Read the model definition and answer for the solid it produces. Units are mm, in the model's axes. Coordinates: 2 decimals unless noted, no trailing zeros. Write each loop counter-clockwise with the first axis right and the second up, starting at its lowest first coordinate (ties: lowest second). Pieces come first, ordered by that corner, then holes. Notation, with made-up numbers: (3.25, 82) - (57.25, 82) arc R9 ccw to (57.25, 93) - close; hole circle Ø9 at (-26, 22.5). An arc over 180 degrees is marked (long way). Return JSON: item names as keys, results as strings.
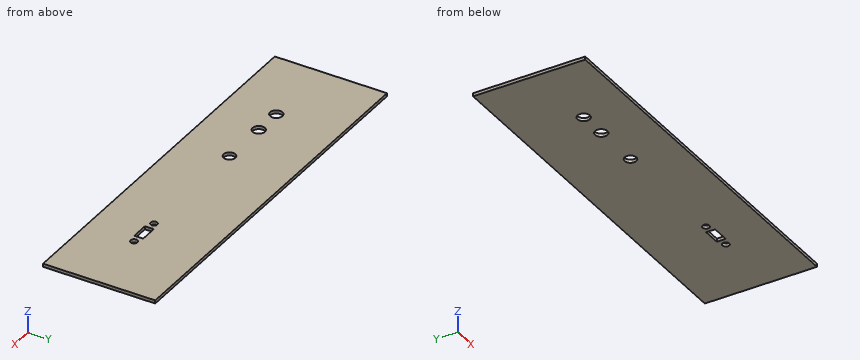
```python
from build123d import *

# Parameters (mm, degrees)
SKETCH_W      = 198
SKETCH_H      = 58
PAD_DEPTH     = 1.65
SKETCH001_R   = 1.75
SKETCH001_R_2 = 3
SKETCH001_R_3 = 3.175
SKETCH001_W   = 9.1
SKETCH001_H   = 4.6
POCKET_DEPTH  = 5


with BuildPart() as part:
    # Sketch → Pad (new body)
    with BuildSketch(Plane.XY):
        with Locations((99, 29)):
            Rectangle(SKETCH_W, SKETCH_H)
    extrude(amount=PAD_DEPTH)

    # Sketch001 (on Face6 of Pad) → Pocket (cut)
    with BuildSketch(Plane.XY.offset(1.65)):
        with Locations((144.5, 25)):
            Circle(SKETCH001_R)
        with Locations((161.5, 25)):
            Circle(SKETCH001_R)
        with Locations((80, 25)):
            Circle(SKETCH001_R_2)
        with Locations((40, 25)):
            Circle(SKETCH001_R_3)
        with Locations((55, 25)):
            Circle(SKETCH001_R_3)
        with Locations((153, 25)):
            Rectangle(SKETCH001_W, SKETCH001_H)
    extrude(amount=-POCKET_DEPTH, mode=Mode.SUBTRACT)


solid = part.part
```
(1) A cutting plane is placed at B-B (y = 25). Determine the outline of the cut face in (x, z) (3 decimals), and give its area (3 significant figures).
Answer:
{"outline": "(0, 0) - (36.825, 0) - (36.825, 1.65) - (0, 1.65) - close; (43.175, 0) - (51.825, 0) - (51.825, 1.65) - (43.175, 1.65) - close; (58.175, 0) - (77, 0) - (77, 1.65) - (58.175, 1.65) - close; (83, 0) - (142.75, 0) - (142.75, 1.65) - (83, 1.65) - close; (146.25, 0) - (148.45, 0) - (148.45, 1.65) - (146.25, 1.65) - close; (157.55, 0) - (159.75, 0) - (159.75, 1.65) - (157.55, 1.65) - close; (163.25, 0) - (198, 0) - (198, 1.65) - (163.25, 1.65) - close", "area": "269 mm²"}
(2) A flat-ended cylindrical pin translates along its axis: P1, Ø9.5, axis at x = 80, y = 25, coming from the +Z side. Find the tip coordinate at first contact, or state that the pin passes through.
Answer:
{"P1": "z = 1.65"}
(3) A cutting plane is placed at A-A (x = 55). Determine the outline of the cut face in (y, z) (3 decimals), and give its area (3 significant figures).
Answer:
{"outline": "(0, 0) - (21.825, 0) - (21.825, 1.65) - (0, 1.65) - close; (28.175, 0) - (58, 0) - (58, 1.65) - (28.175, 1.65) - close", "area": "85.2 mm²"}
(4) A cutting plane is placed at C-C (x = 144.5). Determine the outline of the cut face in (y, z).
Answer:
{"outline": "(0, 0) - (23.25, 0) - (23.25, 1.65) - (0, 1.65) - close; (26.75, 0) - (58, 0) - (58, 1.65) - (26.75, 1.65) - close"}
(5) Straight lines are drawn through the part: line 1 (Y direction, x = 161.5, z = 0.4); line 2 (Y direction, x = 80, z = 0.85); line 3 (X direction, y = 27, z = 0.6). For each, find the intervals that lie inside material, in ascending order. Write a range as from..to.
Answer:
{"line 1": "0..23.25, 26.75..58", "line 2": "0..22, 28..58", "line 3": "0..37.53, 42.47..52.53, 57.47..77.76, 82.24..148.45, 157.55..198"}
